Here's how the part is built. I have some questions about the finished solid (model axes, mm). A direction names the side the tool comes from. Coordinates: 2 decimals unless noted, no trailing zeros. Loops run counter-clockwise (first coordinate to the right, second up) from the corner with the lowest first, then second, coordinate; pieces in that order, holes last.
from build123d import *

# Parameters (mm, degrees)
SKETCH1_R          = 24.95
HUB_DEPTH          = 7
SKETCH2_R          = 27.5
SHOULDER_DEPTH     = 4
SKETCH3_R          = 4
CUT_EXTRUDE1_DEPTH = 41.416580756
SKETCH5_R          = 1.4
CUT_EXTRUDE3_DEPTH = 8
SKETCH6_R          = 3
CUT_EXTRUDE4_DEPTH = 6


with BuildPart() as part:
    # Sketch1 → Hub (new body)
    with BuildSketch(Plane(origin=(0, 0, 0), x_dir=(0, 0, -1), z_dir=(1, 0, 0))):
        Circle(SKETCH1_R)
    extrude(amount=HUB_DEPTH)

    # Sketch2 → Shoulder (add)
    with BuildSketch(Plane(origin=(7, 0, 0), x_dir=(0, 0, -1), z_dir=(1, 0, 0))):
        Circle(SKETCH2_R)
    extrude(amount=SHOULDER_DEPTH)

    # Sketch3 → Cut-Extrude1 (cut, through all)
    with BuildSketch(Plane(origin=(11, 0, 0), x_dir=(0, 0, -1), z_dir=(1, 0, 0))):
        Circle(SKETCH3_R)
    extrude(amount=-CUT_EXTRUDE1_DEPTH, mode=Mode.SUBTRACT)

    # Sketch5 → Cut-Extrude3 (cut)
    with BuildSketch(Plane(origin=(11, 0, 0), x_dir=(0, 0, -1), z_dir=(1, 0, 0))):
        with Locations((-12, 0)):
            Circle(SKETCH5_R)
        with Locations((0, 12)):
            Circle(SKETCH5_R)
        with Locations((12, 0)):
            Circle(SKETCH5_R)
        with Locations((0, -12)):
            Circle(SKETCH5_R)
    extrude(amount=-CUT_EXTRUDE3_DEPTH, mode=Mode.SUBTRACT)

    # Sketch6 → Cut-Extrude4 (cut)
    with BuildSketch(Plane.ZY):
        with Locations((0, 20)):
            Circle(SKETCH6_R)
        with Locations((18.186533479, 10.5)):
            Circle(SKETCH6_R)
        with Locations((19.052558883, -10)):
            Circle(SKETCH6_R)
        with Locations((1.732050808, -21)):
            Circle(SKETCH6_R)
        with Locations((-16.454482672, -11.5)):
            Circle(SKETCH6_R)
        with Locations((-17.320508076, 9)):
            Circle(SKETCH6_R)
    extrude(amount=-CUT_EXTRUDE4_DEPTH, mode=Mode.SUBTRACT)


solid = part.part
Q1. Suppose I cut it at D-D on x = 5.25. State how many separate pieces and enclosed holes the cut face has, and give its area (3 significant figures).
Q2. For faces 1 (the cylindrical face through (7.06, -10.82, -0.75)), 2 (the cylindrical face through (5.577, -3.905, 0.867)), 3 (the cylindrical face through (2.96, -11.37, -19.45)), which set-ups out of +Z, -Z, +X, -X, +Y, -Y let a thin tool reach every point of the face, with its end or its side?
Q3. Please list where these lines run through material, in increasing order: probe 1 along Y at (x, z) = (1.5, -17); probe 2 along Y at (x, z) = (5.5, 0); probe 3 along X at (y, z) = (4, 25).
Q4. Suppose I cut it at B-B on x = 1.75. Write out the boundary of the cut face in (y, z), and give its area (3 significant figures).
Q5. We'd pull the mould along Y, two halves only. Please class faces 4 (the flat face through (0, -5, 0)), 5 (the cylindrical face through (8.972, -26.846, 5.961)), 6 (the flat face through (3, -12, 0)): pulls with the +Y half, pulls with the -Y half, needs draft (parallel to the pull), parting line crosses it, or undercut.
Q6. Suppose I cut it at A-A on y = 0. Write out the boundary of the cut face in (x, z), and give its area (4 significant figures).
Q7. Suppose I cut it at C-C on z = 0. Write out the boundary of the cut face in (x, y), and give its area (3 significant figures).
Q8. Will these pins go through, and if not, where does the flat tip stop? P1, Ø2, axis at x = 9.5, y = 15, coming from the +Z side; P2, Ø1, axis at y = -17.5, z = 19, coming from the -X side; P3, Ø3, axis at x = 8.5, y = -7, coming from the -Z side.
Check values:
1. separate pieces: 1
1. enclosed holes: 11
1. area: 1,710 mm2
2. face 1: +X
2. face 2: +X, -X
2. face 3: -X
3. probe 1: y = -18.26 to -14.45, -8.55 to 6.02, 11.98 to 18.26
3. probe 2: y = -24.95 to -23.45, -18.55 to -13.4, -10.6 to -4, 4 to 10.6, 13.4 to 17, 23 to 24.95
3. probe 3: x = 7 to 11
4. outline: circle Ø49.9 at (0, 0); hole circle Ø6 at (-21, 1.73); hole circle Ø6 at (-11.5, -16.45); hole circle Ø6 at (-10, 19.05); hole circle Ø8 at (0, 0); hole circle Ø6 at (9, -17.32); hole circle Ø6 at (10.5, 18.19); hole circle Ø6 at (20, 0)
4. area: 1,740 mm2
5. face 4: needs draft
5. face 5: parting line crosses it
5. face 6: undercut
6. outline: (0, -24.95) - (7, -24.95) - (7, -27.5) - (11, -27.5) - (11, -13.4) - (3, -13.4) - (3, -10.6) - (11, -10.6) - (11, -4) - (0, -4) - close; (0, 4) - (11, 4) - (11, 10.6) - (3, 10.6) - (3, 13.4) - (11, 13.4) - (11, 27.5) - (7, 27.5) - (7, 24.95) - (0, 24.95) - close
6. area: 436.5 mm2
7. outline: (0, -24.95) - (7, -24.95) - (7, -27.5) - (11, -27.5) - (11, -13.4) - (3, -13.4) - (3, -10.6) - (11, -10.6) - (11, -4) - (0, -4) - (0, -18.55) - (6, -18.55) - (6, -23.45) - (0, -23.45) - close; (0, 4) - (11, 4) - (11, 10.6) - (3, 10.6) - (3, 13.4) - (11, 13.4) - (11, 27.5) - (7, 27.5) - (7, 24.95) - (0, 24.95) - (0, 23) - (6, 23) - (6, 17) - (0, 17) - close
7. area: 371 mm2
8. P1: stops at z = 23.67
8. P2: stops at x = 7
8. P3: stops at z = -26.94
